For this review, take the finished solid that the model builds, in its own axes (mm). Face numbers are marked on the shaded views. A direction names the side the tool comes from. Round coordinates to 2 decimals unless told otherwise and drop trailing zeros. Order: outer loops, then holes, each group sorted by start corner. A loop starts at its lowest first (then second) coordinate and runs counter-clockwise, first axis right, second up. Notation, with made-up numbers: (77.25, -33.75) - (117.25, -33.75) arc R10 cw to (117.25, -26.75) - close; hole circle Ø8 at (25, 88.5). An arc over 180 degrees is marked (long way). One line per question, with ' | ' between items.
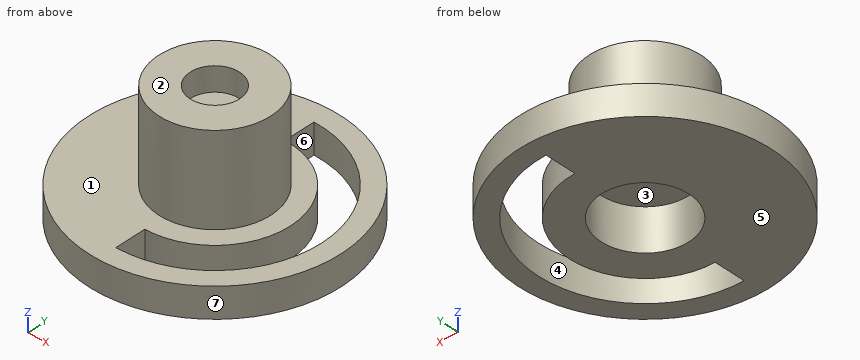
Solid Edge part; units mm, degrees
sketch "Sketch1" plane through (0, 0, 0) normal (0, 0, 1) x (1, 0, 0)
  circle A0 centre (0, 0) radius 4.65
extrude "Protrusion1" add sketch "Sketch1" along normal blind 10
sketch "Sketch2" plane through (0, 0, 10) normal (0, 0, 1) x (1, 0, 0)
  circle A0 centre (0, 0) radius 2.05
extrude "VaciadoExtruido_1" cut sketch "Sketch2" against normal blind 2
sketch "Sketch3" plane through (0, 0, 0) normal (0, 0, -1) x (1, 0, 0)
  circle A0 centre (0, 0) radius 3.65
extrude "VaciadoExtruido_2" cut sketch "Sketch3" against normal blind 3.5
extrude "ProtrusiónExtruida_2" [suppressed]
sketch "Sketch4" plane through (0, 0, 0) normal (0, 0, -1) x (0, 1, 0)
  circle A0 centre (0, 0) radius 10.5
  circle A1 centre (0, 0) radius 4.65
extrude "Protrusion2" add sketch "Sketch4" against normal blind 2.5
sketch "Sketch5" plane through (0, 0, 0) normal (1, 0, 0) x (0, 1, 0)
  line L0 (8.875, 0) -> (6.275, 0)
  line L1 (6.275, 0) -> (6.275, 2.5)
  line L2 (6.275, 2.5) -> (8.875, 2.5)
  line L3 (8.875, 2.5) -> (8.875, 0)
revolve "VaciadoPorRevolución_2" cut sketch "Sketch5" angle 180 about axis through (0, 0, 0) along (0, 0, -1)
(1) Insertion check: pin 1 (5 mm diameter, centred on x = 7.5, z = 2.5, fed in from +Y); pin 2 (1.5 mm diameter, centred on y = 7, z = 6, fed in from -X); pin 3 (4 mm diameter, centred on x = -6, y = -3, fed in from +Z); pin 4 (4 mm diameter, centred on x = -0.5, y = -0.5, fed in from -Z). Each pin has a flat end and moves straight along its axis. Give the tip position at first contact, or say it passes through.
Output values:
pin 1: y = 9.23 | pin 2: through | pin 3: z = 2.5 | pin 4: z = 3.5
(2) We need section A-A on y = 0. State the section outline as (x, z) points (3 decimals).
Output values:
outline: (-10.5, 0) - (-3.65, 0) - (-3.65, 3.5) - (3.65, 3.5) - (3.65, 0) - (6.275, 0) - (6.275, 2.5) - (4.65, 2.5) - (4.65, 10) - (2.05, 10) - (2.05, 8) - (-2.05, 8) - (-2.05, 10) - (-4.65, 10) - (-4.65, 2.5) - (-10.5, 2.5) - close; (8.875, 0) - (10.5, 0) - (10.5, 2.5) - (8.875, 2.5) - close
(3) We need section D-D on z = 7.5. State the section outline as (x, y) points, plus the area to 3 significant figures.
Output values:
outline: circle Ø9.3 at (0, 0) | area: 67.9 mm^2
(4) Mouldability with a two-part tool opening along Y and no side actions: class the marked faces 5, 6 and 7 as released by +Y, released by -Y, zero draft, split by the parting line, or undercut.
Output values:
face 5: zero draft | face 6: undercut | face 7: split by the parting line
(5) For the marked faces 1, 2, 3 and 4, list the 3-axis set-ups (+Z, -Z, +X, -X, +Y, -Y) from which the entire face can be reached by the end or side of a thin tool; tool diameter is ignored.
Output values:
face 1: +Z | face 2: +Z, +X, -X, +Y, -Y | face 3: -Z | face 4: +Z, -Z
(6) We need section B-B on x = 6.75. State the section outline as (y, z) points.
Output values:
outline: (-8.04, 0) - (-5.76, 0) - (-5.76, 2.5) - (-8.04, 2.5) - close; (5.76, 0) - (8.04, 0) - (8.04, 2.5) - (5.76, 2.5) - close
(7) For probe 1 along Y at (x, z) = (0, 9.3); probe 2 along Y at (x, z) = (0, 2.75); probe 3 along X at (y, z) = (0, 2.15) (3 decimals), list the stretches that pass through material, from the lowest coordinate up. Write a range as [from, to].
Output values:
probe 1: [-4.65, -2.05], [2.05, 4.65] | probe 2: [-4.65, -3.65], [3.65, 4.65] | probe 3: [-10.5, -3.65], [3.65, 6.275], [8.875, 10.5]
(8) We need section C-C on z = 1. State the section outline as (x, y) points (3 decimals), plus the area to 3 significant figures.
Output values:
outline: circle Ø21 at (0, 0); hole circle Ø7.3 at (0, 0); hole (0, -8.875) arc R8.875 ccw to (0, 8.875) - (0, 6.275) arc R6.275 cw to (0, -6.275) - close | area: 243 mm^2
